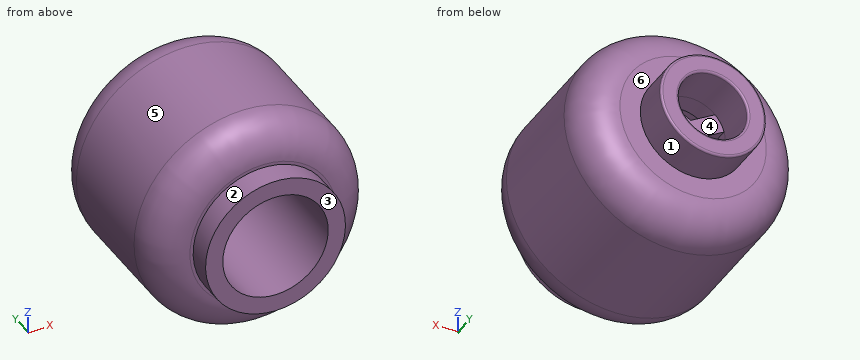
from build123d import *

# Parameters (mm, degrees)
CROQUIS3_R            = 1.6
CORTAR_EXTRUIR1_DEPTH = 2
CORTAR_EXTRUIR2_DEPTH = 0.9
MATRIZC1_COUNT        = 3
REDONDEO1_R           = 0.1


with BuildPart() as part:
    # Croquis1 → Revolución1 (revolve)
    with BuildSketch(Plane(origin=(0, 0, 0), x_dir=(0, 0, -1), z_dir=(1, 0, 0))):
        with BuildLine():
            Line((2.45, 0), (3.25, 0))
            Line((3.25, 0), (3.25, 1.1))
            Line((3.25, 1.1), (3.4, 1.1))
            ThreePointArc((3.4, 1.1), (4.602082, 1.597918), (5.1, 2.8))
            Line((5.1, 2.8), (5.1, 7.9))
            ThreePointArc((5.1, 7.9), (4.602082, 9.102082), (3.4, 9.6))
            Line((3.4, 9.6), (2.45, 9.6))
            Line((2.45, 9.6), (2.45, 11.4))
            Line((2.45, 11.4), (0, 11.4))
            Line((0, 11.4), (0, 8.5))
            Line((0, 8.5), (2.45, 8.5))
            Line((2.45, 8.5), (2.45, 0))
        make_face()
    revolve(axis=Axis((0, 0, 0), (0, 1, 0)))

    # Croquis3 → Cortar-Extruir1 (cut)
    with BuildSketch(Plane(origin=(0, 11.4, 0), x_dir=(1, 0, 0), z_dir=(0, 1, 0))):
        Circle(CROQUIS3_R)
    extrude(amount=-CORTAR_EXTRUIR1_DEPTH, mode=Mode.SUBTRACT)

    # Croquis4 → Cortar-Extruir2 (cut)
    with BuildSketch(Plane(origin=(0, 9.4, 0), x_dir=(1, 0, 0), z_dir=(0, 1, 0))):
        with BuildLine():
            Line((-1.547049, -0.408215), (-0.42, 0.242487))
            Line((-0.42, 0.242487), (-0.42, 1.543891))
            ThreePointArc((-0.42, 1.543891), (-1.385641, 0.8), (-1.547049, -0.408215))
        make_face()
    cortar_extruir2 = extrude(amount=-CORTAR_EXTRUIR2_DEPTH, mode=Mode.SUBTRACT)

    # MatrizC1: Cortar-Extruir2 ×3 about axis
    matrizc1_axis = Axis((0, 0, 0), (0, 1, 0))
    for i in range(1, MATRIZC1_COUNT):
        add(cortar_extruir2.rotate(matrizc1_axis, i * 360 / MATRIZC1_COUNT), mode=Mode.SUBTRACT)

    # Redondeo1
    redondeo1_edges = [part.edges().sort_by_distance(p)[0] for p in [
        (-1.6, 11.4, 0),
        (0, 11.4, 2.45),
    ]]
    fillet(redondeo1_edges, radius=REDONDEO1_R)


solid = part.part
Build history of the part. All positions in model axes, mm. Face numbers are marked on the shaded views. A direction names the side the tool comes from. Coordinates: 2 decimals unless noted, no trailing zeros. Write each loop counter-clockwise with the first axis right and the second up, starting at its lowest first coordinate (ties: lowest second). Pieces come first, ordered by that corner, then holes. Notation, with made-up numbers: (83, 65.25) -> (129, 65.25) arc R36 cw to (129, 101.25) -> close; hole circle Ø1 at (-34.5, 86). An arc over 180 degrees is marked (long way). Use CSV: the item, a comma, the result in double quotes. Start each with the question number.
Q1. 3-axis set-ups, long thin cutter, end or side, ignore diameter. For the marked faces 1, 2 and 3: which of +Z, -Z, +X, -X, +Y, -Y reach the whole face in a straight line?
Q2. Cut at B-B, the plane y = 10.75. List the corners of the cut face in (x, z).
Q3. Drill centre lines: probe 1 along Z at (x, y) = (0, 9.9); probe 2 along X at (y, z) = (6.5, 0). Where is each one in solid material? Low to high.
Q4. Pull direction Z, two halves, no side cores. Call the marked faces 4, 5 and 6: released by +Z, released by -Z, zero draft, split by the parting line, or undercut.
Q5. Cut at C-C, the plane y = 4.5. List the corners of the cut face in (x, z), then the cut area to 3 significant figures.
Q6. Cut at A-A, the plane z = 0. State how many separate pieces and enclosed holes the cut face has, then the cut area to 3 significant figures.
Q7. Flat gauge pins, fed straight in: pin 1 Ø1 at (y, z) = (9, -1) entering from -X; pin 2 Ø1.5 at (x, y) = (-1.5, 1.5) entering from +Z; pin 3 Ø5 at (x, y) = (3.5, 5) entering from -Z. Where does each tip first touch, or does it go through?
Checked values:
1,face 1,"+Y"
1,face 2,"-Y"
1,face 3,"+Z, -Z, +X, -X, -Y"
2,outline,"circle Ø4.9 at (0, 0); hole circle Ø3.2 at (0, 0)"
3,probe 1,"z = -2.45 to -1.6, 1.6 to 2.45"
3,probe 2,"x = -5.1 to -2.45, 2.45 to 5.1"
4,face 4,"undercut"
4,face 5,"split by the parting line"
4,face 6,"zero draft"
5,outline,"circle Ø10.2 at (0, 0); hole circle Ø4.9 at (0, 0)"
5,area,"62.9 mm²"
6,separate pieces,"3"
6,enclosed holes,"0"
6,area,"50.8 mm²"
7,pin 1,"stops at x = -4.91"
7,pin 2,"stops at z = 4.84"
7,pin 3,"stops at z = -5"
